For this review, use the dimensioned drawing (mm, ordinates from the lowest corner) and the shaded views. A direction names the side the tool comes from. Round coordinates to 2 decimals unless told otherwise and drop trailing zeros. Order: outer loops, then holes, each group sorted by start corner. A loop starts at its lowest first (then second) coordinate and runs counter-clockwise, first axis right, second up. Notation, with made-up numbers: M -19,-39.5 L 38,-39.5 A12 cw 38,-31.5 Z; hole C 24,-9 d6. An arc over 180 degrees is marked long. Use a Markdown table: item, result. Add a question column.
1. Consider section C-C on x = 13.25. State the section outline as (y, z) points.
2. Consider section B-B on y = 13. State the section outline as (x, z) points (1 decimal).
3. Consider section A-A on z = 3.25. State the section outline as (x, y) points (1 decimal), then the cut area to 3 significant figures.
4. To check wall thickness, follow probe 1 along Z at (x, y) = (15.25, 6.75); probe 2 along Y at (x, z) = (5.5, 1.8); probe 3 along X at (y, z) = (9.5, 0.7) (1 decimal). State the ranges of each line that lie inside material, in increasing order.
5. For the marked faces 1, 2, 3 and 4, list the 3-axis set-ups (+Z, -Z, +X, -X, +Y, -Y) from which the entire face can be reached by the end or side of a thin tool; tool diameter is ignored.
6. Insertion check: P1, Ø1.4, axis at x = 22, y = 9.5, coming from the +Z side; P2, Ø6.5, axis at x = 16, y = 3.5, coming from the -Z side; P3, Ø8, axis at x = 17, y = 17, coming from the -Z side; P4, Ø2, axis at x = 6.5, z = 2.5, coming from the +Y side. Each pin has a flat end and moves straight along its axis. Give the tip position at first contact, or say it passes through.
7. Consider section D-D on y = 16. State the section outline as (x, z) points.
8. The part is to be moulded in two halves that separate along X. For the marked faces 5, 6 and 7, say which applies: +X half, -X half, draft (parallel to the pull), parting line (faces both ways), or undercut.
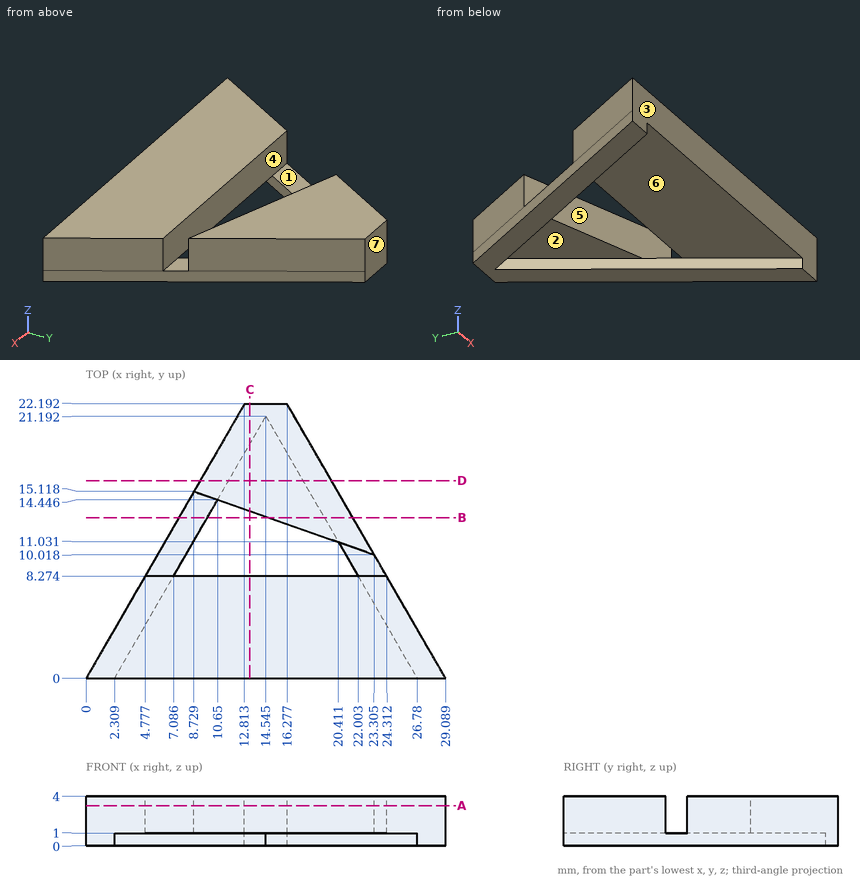
Answer block:
| question | item | result |
|---|---|---|
| 1 | outline | M 0,1 L 8.27,1 L 8.27,4 L 0,4 Z; M 13.54,1 L 18.95,1 L 18.95,0 L 22.19,0 L 22.19,4 L 13.54,4 Z |
| 2 | outline | M 7.5,0 L 9.8,0 L 9.8,1 L 7.5,1 Z; M 14.8,1 L 19.3,1 L 19.3,0 L 21.6,0 L 21.6,4 L 14.8,4 Z |
| 3 | outline | M 0,0 L 29.1,0 L 24.3,8.3 L 4.8,8.3 Z; M 8.7,15.1 L 23.3,10 L 16.3,22.2 L 12.8,22.2 Z |
| 3 | area | 284 mm^2 |
| 4 | probe 1 | 1 to 4 |
| 4 | probe 2 | 0 to 8.27 |
| 4 | probe 3 | 5.5 to 7.8, 21.3 to 23.6 |
| 5 | face 1 | +Z, -X |
| 5 | face 2 | -Z, -Y |
| 5 | face 3 | +Z, -Z, +X, -X, -Y |
| 5 | face 4 | +Z, +X, -X |
| 6 | P1 | z = 1 |
| 6 | P2 | z = 1 |
| 6 | P3 | z = 0 |
| 6 | P4 | y = 8.27 |
| 7 | outline | M 9.24,0 L 11.55,0 L 11.55,1 L 17.54,1 L 17.54,0 L 19.85,0 L 19.85,4 L 9.24,4 Z |
| 8 | face 5 | -X half |
| 8 | face 6 | undercut |
| 8 | face 7 | draft |
